from build123d import *

# Parameters (mm, degrees)
SKETCH1_W                   = 100
SKETCH1_H                   = 10
BOSS_EXTRUDE1_DEPTH         = 15
SKETCH2_R                   = 7.5
BOSS_EXTRUDE2_DEPTH         = 30
SKETCH3_W                   = 18.5
SKETCH3_H                   = 18.5
BOSS_EXTRUDE3_DEPTH         = 20
CHAMFER1_SIZE               = 3
CHAMFER2_SIZE               = 5
SKETCH4_W                   = 11.2
SKETCH4_H                   = 5.65
CUT_EXTRUDE1_DEPTH          = 121.694863188
F_1_4_CLEARANCE_HOLE1_D     = 7.14248
F_1_4_CLEARANCE_HOLE1_DEPTH = 25
F_1_4_CLEARANCE_HOLE1_TIP   = 2.145817477
SKETCH8_W                   = 15
SKETCH8_H                   = 15
BOSS_EXTRUDE4_DEPTH         = 5
SKETCH9_R                   = 2.65
CUT_EXTRUDE2_DEPTH          = 25
F_4_CLEARANCE_HOLE1_D       = 3.4544
F_4_CLEARANCE_HOLE1_DEPTH   = 10
F_4_CLEARANCE_HOLE1_TIP     = 1.037806461
SKETCH13_W                  = 6.6
SKETCH13_H                  = 2.79
CUT_EXTRUDE3_DEPTH          = 7.7559
SKETCH14_W                  = 15
SKETCH14_H                  = 15
BOSS_EXTRUDE5_DEPTH         = 3
SKETCH15_W                  = 2.5
SKETCH15_H                  = 15
CUT_EXTRUDE4_DEPTH          = 42.5
SKETCH16_W                  = 2.5
SKETCH16_H                  = 15
CUT_EXTRUDE5_DEPTH          = 42.5


with BuildPart() as part:
    # Sketch1 → Boss-Extrude1 (new body)
    with BuildSketch(Plane(origin=(0, 0, 0), x_dir=(1, 0, 0), z_dir=(0, 1, 0))):
        with Locations((50, 5)):
            Rectangle(SKETCH1_W, SKETCH1_H)
    extrude(amount=BOSS_EXTRUDE1_DEPTH)

    # Sketch2 → Boss-Extrude2 (add)
    with BuildSketch(Plane(origin=(0, 15, 0), x_dir=(1, 0, 0), z_dir=(0, 1, 0))):
        with Locations(Location((50, 5, 0), (0, 0, 41.810314896))):
            Circle(SKETCH2_R)
    extrude(amount=BOSS_EXTRUDE2_DEPTH)

    # Sketch3 → Boss-Extrude3 (add)
    with BuildSketch(Plane(origin=(0, 45, 0), x_dir=(1, 0, 0), z_dir=(0, 1, 0))):
        with Locations((50, 5)):
            Rectangle(SKETCH3_W, SKETCH3_H)
    extrude(amount=BOSS_EXTRUDE3_DEPTH)

    # Chamfer1
    chamfer1_edges = [part.edges().sort_by_distance(p)[0] for p in [
        (40.75, 65, -5),
        (50, 65, 4.25),
        (59.25, 65, -5),
        (50, 65, -14.25),
    ]]
    chamfer(chamfer1_edges, length=CHAMFER1_SIZE)

    # Chamfer2
    # the kernel refuses this chamfer: 5 mm, written as the material it takes off along each edge
    with BuildSketch(Plane(origin=(27.89158506, 45, -14.25), x_dir=(0, 0.9996219169112968, -0.027495876610586317), z_dir=(1, 0, 0))) as chamfer2_piece_1_section:
        Polygon((CHAMFER2_SIZE * 0.999621916911, CHAMFER2_SIZE * 0.0274958766106), (-CHAMFER2_SIZE * 0.0274958766106, CHAMFER2_SIZE * 0.999621916911), (0, 0), align=None)
    chamfer2_piece_1 = extrude(amount=44.21682988, mode=Mode.PRIVATE)
    chamfer2_piece_1 = chamfer2_piece_1 - Plane(origin=(50, 46.70985324, -5), x_dir=(0.7453559924973537, 0, -0.6666666666695469), z_dir=(0, -1, 0)) * Cylinder(7.5, 109, mode=Mode.PRIVATE)
    with BuildSketch(Plane(origin=(40.75, 45, 17.10841494), x_dir=(-0.027495876610586317, 0.9996219169112968, 0), z_dir=(0, 0, -1))) as chamfer2_piece_2_section:
        Polygon((CHAMFER2_SIZE * 0.999621916911, CHAMFER2_SIZE * 0.0274958766106), (-CHAMFER2_SIZE * 0.0274958766106, CHAMFER2_SIZE * 0.999621916911), (0, 0), align=None)
    chamfer2_piece_2 = extrude(amount=44.21682988, mode=Mode.PRIVATE)
    chamfer2_piece_2 = chamfer2_piece_2 - Plane(origin=(50, 46.709853278, -5), x_dir=(0.7453559924973537, 0, -0.6666666666695469), z_dir=(0, -1, 0)) * Cylinder(7.5, 109, mode=Mode.PRIVATE)
    with BuildSketch(Plane(origin=(59.25, 45, -27.10841494), x_dir=(-0.9996219169112968, -0.027495876610586317, 0), z_dir=(0, 0, 1))) as chamfer2_piece_3_section:
        Polygon((CHAMFER2_SIZE * 0.999621916911, -CHAMFER2_SIZE * 0.0274958766106), (-CHAMFER2_SIZE * 0.0274958766106, -CHAMFER2_SIZE * 0.999621916911), (0, 0), align=None)
    chamfer2_piece_3 = extrude(amount=44.21682988, mode=Mode.PRIVATE)
    chamfer2_piece_3 = chamfer2_piece_3 - Plane(origin=(50, 46.709853248, -5), x_dir=(0.7453559924973537, 0, -0.6666666666695469), z_dir=(0, -1, 0)) * Cylinder(7.5, 109, mode=Mode.PRIVATE)
    with BuildSketch(Plane(origin=(72.10841494, 45, 4.25), x_dir=(0, -0.027495876610586317, -0.9996219169112968), z_dir=(-1, 0, 0))) as chamfer2_piece_4_section:
        Polygon((CHAMFER2_SIZE * 0.999621916911, -CHAMFER2_SIZE * 0.0274958766106), (-CHAMFER2_SIZE * 0.0274958766106, -CHAMFER2_SIZE * 0.999621916911), (0, 0), align=None)
    chamfer2_piece_4 = extrude(amount=44.21682988, mode=Mode.PRIVATE)
    chamfer2_piece_4 = chamfer2_piece_4 - Plane(origin=(50, 46.709853226, -5), x_dir=(0.7453559924973537, 0, -0.6666666666695469), z_dir=(0, -1, 0)) * Cylinder(7.5, 109, mode=Mode.PRIVATE)
    add([chamfer2_piece_1, chamfer2_piece_2, chamfer2_piece_3, chamfer2_piece_4], mode=Mode.SUBTRACT)

    # Sketch4 → Cut-Extrude1 (cut, through all)
    with BuildSketch(Plane.XY.offset(4.25)):
        with Locations((50, 56)):
            Rectangle(SKETCH4_W, SKETCH4_H)
    extrude(amount=-CUT_EXTRUDE1_DEPTH, mode=Mode.SUBTRACT)

    # 1/4 Clearance Hole1
    with Locations(Plane(origin=(0, 65, 0), x_dir=(1, 0, 0), z_dir=(0, 1, 0))):
        with Locations((50, 5)):
            Hole(F_1_4_CLEARANCE_HOLE1_D / 2, depth=F_1_4_CLEARANCE_HOLE1_DEPTH)
            with Locations((0, 0, -(F_1_4_CLEARANCE_HOLE1_DEPTH + F_1_4_CLEARANCE_HOLE1_TIP / 2))):  # 118° drill point
                Cone(0, F_1_4_CLEARANCE_HOLE1_D / 2, F_1_4_CLEARANCE_HOLE1_TIP, mode=Mode.SUBTRACT)

    # Sketch8 → Boss-Extrude4 (add)
    with BuildSketch(Plane.XY):
        with Locations((50, 7.5)):
            Rectangle(SKETCH8_W, SKETCH8_H)
    extrude(amount=BOSS_EXTRUDE4_DEPTH)

    # Sketch9 → Cut-Extrude2 (cut)
    with BuildSketch(Plane.XZ):
        with Locations(Location((50, -5, 0), (0, 0, 270))):
            Circle(SKETCH9_R)
    extrude(amount=-CUT_EXTRUDE2_DEPTH, mode=Mode.SUBTRACT)

    # #4 Clearance Hole1
    with Locations(Plane.XY.offset(5)):
        with Locations((50, 5)):
            Hole(F_4_CLEARANCE_HOLE1_D / 2, depth=F_4_CLEARANCE_HOLE1_DEPTH)
            with Locations((0, 0, -(F_4_CLEARANCE_HOLE1_DEPTH + F_4_CLEARANCE_HOLE1_TIP / 2))):  # 118° drill point
                Cone(0, F_4_CLEARANCE_HOLE1_D / 2, F_4_CLEARANCE_HOLE1_TIP, mode=Mode.SUBTRACT)

    # Sketch13 → Cut-Extrude3 (cut)
    with BuildSketch(Plane.XZ):
        with Locations((50, 1.105)):
            Rectangle(SKETCH13_W, SKETCH13_H)
    extrude(amount=-CUT_EXTRUDE3_DEPTH, mode=Mode.SUBTRACT)

    # Sketch14 → Boss-Extrude5 (add)
    with BuildSketch(Plane(origin=(0, 0, -10), x_dir=(-1, 0, 0), z_dir=(0, 0, -1))):
        with Locations((-50, 7.5)):
            Rectangle(SKETCH14_W, SKETCH14_H)
    extrude(amount=BOSS_EXTRUDE5_DEPTH)

    # Sketch15 → Cut-Extrude4 (cut)
    with BuildSketch(Plane(origin=(100, 0, 0), x_dir=(0, 0, -1), z_dir=(1, 0, 0))):
        with Locations((1.25, 7.5)):
            Rectangle(SKETCH15_W, SKETCH15_H)
        with Locations((8.75, 7.5)):
            Rectangle(SKETCH15_W, SKETCH15_H)
    extrude(amount=-CUT_EXTRUDE4_DEPTH, mode=Mode.SUBTRACT)

    # Sketch16 → Cut-Extrude5 (cut)
    with BuildSketch(Plane.ZY):
        with Locations((-8.75, 7.5)):
            Rectangle(SKETCH16_W, SKETCH16_H)
        with Locations((-1.25, 7.5)):
            Rectangle(SKETCH16_W, SKETCH16_H)
    extrude(amount=-CUT_EXTRUDE5_DEPTH, mode=Mode.SUBTRACT)


solid = part.part
Design review of the part built by this model. Coordinates are the model's own, in mm. A direction names the side the tool comes from. Coordinates: 2 decimals unless noted, no trailing zeros. Order: outer loops, then holes, each group sorted by start corner. A loop starts at its lowest first (then second) coordinate and runs counter-clockwise, first axis right, second up.
Item 1: For line 1 (Z direction, x = 50, y = 14.25); line 2 (Z direction, x = 50, y = 46); line 3 (Z direction, x = 38.5, y = 5.5), list the stretches that pass through material, from the lowest coordinate up.
Item 2: For faces 4 (the flat face through (46, 53.175, -5)), 5 (the flat face through (50, 3, -0.29)), 6 (the flat face through (59.25, 56, -5)), list the 3-axis set-ups (+Z, -Z, +X, -X, +Y, -Y) from which the entire face can be reached by the end or side of a thin tool; tool diameter is ignored.
Item 3: Take a section at C-C, the plane y = 20. Write out the cut boundary in (x, z).
Item 4: Take a section at A-A, the plane y = 5. Write out the cut boundary in (x, z), then the cut area to 3 significant figures.
Item 5: The part is to be moulded in two halves that separate along X. For faces 1 (the flat face through (0, 7, -5)), 2 (the flat face through (53, 65, -2)), 3 (the cylindrical face through (48.405, 4.338, 3.732)), say which applies: pulls with the +X half, pulls with the -X half, needs draft (parallel to the pull), parting line crosses it, or undercut.
Item 6: For pin 1 Ø8 at (y, z) = (14.5, -12) entering from +X; pin 2 Ø4.5 at (y, z) = (7, -9) entering from -X; pin 3 Ø2 at (y, z) = (4.5, 1) entering from -X; pin 4 Ø7.5 at (x, y) = (49, 3.5) entering from -Z, all flat-tipped, find the tip position at first contact; note any pin that passes through.
Item 7: Take a section at B-B, the plane x = 65.5. Write out the cut boundary in (y, z).
Item 8: Take a section at D-D, the plane y = 34.5. Write out the cut boundary in (x, z).
The answers:
1. line 1: z = -13 to -7.65, -2.35 to 5
1. line 2: z = -12.5 to -8.57, -1.43 to 2.5
1. line 3: z = -7.5 to -2.5
2. face 4: +Z, -Z
2. face 5: -Y
2. face 6: +Z, -Z, +X, +Y
3. outline: circle Ø15 at (50, -5); hole circle Ø5.3 at (50, -5)
4. outline: (0, -7.5) - (42.5, -7.5) - (42.5, -13) - (57.5, -13) - (57.5, -7.5) - (100, -7.5) - (100, -2.5) - (57.5, -2.5) - (57.5, 5) - (51.73, 5) - (51.73, 2.5) - (53.3, 2.5) - (53.3, -0.29) - (51.73, -0.29) - (51.73, -2.99) arc R2.65 cw (long way) to (48.27, -2.99) - (48.27, -0.29) - (46.7, -0.29) - (46.7, 2.5) - (48.27, 2.5) - (48.27, 5) - (42.5, 5) - (42.5, -2.5) - (0, -2.5) - close
4. area: 638 mm2
5. face 1: pulls with the -X half
5. face 2: needs draft
5. face 3: undercut
6. pin 1: stops at x = 57.5
6. pin 2: stops at x = 0
6. pin 3: stops at x = 42.5
6. pin 4: stops at z = -13
7. outline: (0, -7.5) - (15, -7.5) - (15, -2.5) - (0, -2.5) - close
8. outline: circle Ø15 at (50, -5)
